Verification items for the finished model (mm, model axes). Round coordinates to 2 decimals unless told otherwise and drop trailing zeros. Loops run counter-clockwise (first coordinate to the right, second up) from the corner with the lowest first, then second, coordinate; pieces in that order, holes last. Notation, with made-up numbers: (-21.5, -24.5) -> (-1.5, -24.5) arc R25 cw to (-1.5, -7.5) -> close; hole circle Ø10 at (54.5, 51). An arc over 180 degrees is marked (long way). Write item = value, one per line. Start each with the question number.
```python
from build123d import *

# Parameters (mm, degrees)
F0_R     = 292.1
F1_DEPTH = 38.1


with BuildPart() as f1:
    # F0 (on Top) → F1 (new body)
    with BuildSketch(Plane.XY):
        with BuildLine():
            Line((762, 0), (-762, 0))
            Line((-762, 0), (-762, -635))
            ThreePointArc((-762, -635), (-724.802561, -724.802561), (-635, -762))
            Line((-635, -762), (635, -762))
            ThreePointArc((635, -762), (724.802561, -724.802561), (762, -635))
            Line((762, -635), (762, 0))
        make_face()
        with Locations((-342.9, -355.6)):
            Circle(F0_R, mode=Mode.SUBTRACT)
    extrude(amount=-F1_DEPTH)


solid = f1.part
```
(1) Scan lines: line 1 (X direction, y = -362, z = -32.5); line 2 (Y direction, x = -342.9, z = -8.5); line 3 (X direction, y = -355, z = -24). Record each from-to range of solid material in increasing order. Write a range as [from, to].
(2) Section check B-B on y = -355.6. Enter the section's corners in (x, z), then the cut area to 3 significant figures.
(3) Section check C-C on z = -12. Enter the section's corners in (x, y).
(4) Draft check along X on faces 1 (the cylindrical face through (-725.785, -723.81, -18.783)), 2 (the cylindrical face through (-406.222, -640.754, -18.783)), 3 (the flat face through (159, -376, 0)), 4 (the cylindrical face through (723.81, -725.785, -18.783)). Enter one of: +X half, -X half, draft (parallel to the pull), parting line (faces both ways), or undercut.
(5) Section check A-A on x = -342.9. Enter the section's corners in (y, z).
Computed values:
q1.line_1 = [-762, -634.93], [-50.87, 762]
q1.line_2 = [-762, -647.7], [-63.5, 0]
q1.line_3 = [-762, -635], [-50.8, 762]
q2.outline = (-762, -38.1) -> (-635, -38.1) -> (-635, 0) -> (-762, 0) -> close; (-50.8, -38.1) -> (762, -38.1) -> (762, 0) -> (-50.8, 0) -> close
q2.area = 35,800 mm²
q3.outline = (-762, -635) arc R127 ccw to (-635, -762) -> (635, -762) arc R127 ccw to (762, -635) -> (762, 0) -> (-762, 0) -> close; hole circle Ø584.2 at (-342.9, -355.6)
q4.face_1 = -X half
q4.face_2 = undercut
q4.face_3 = draft
q4.face_4 = +X half
q5.outline = (-762, -38.1) -> (-647.7, -38.1) -> (-647.7, 0) -> (-762, 0) -> close; (-63.5, -38.1) -> (0, -38.1) -> (0, 0) -> (-63.5, 0) -> close
